```python
from build123d import *

# Parameters (mm, degrees)
SKETCH3_W          = 81.788
SKETCH3_H          = 40.894
SKETCH3_W_2        = 40.894
SKETCH3_H_2        = 15.748
CUT_EXTRUDE1_DEPTH = 4.7752


with BuildPart() as part:
    # Sketch1 → Revolve1 (revolve)
    with BuildSketch(Plane.XY):
        Polygon((0, 0), (0, 8.90905), (0.762, 9.67105), (4.0386, 9.67105), (4.8006, 8.90905), (5.5626, 8.90905), (5.5626, 10.2235), (13.4874, 10.2235), (13.4874, 0), align=None)
    revolve(axis=Axis((13.4874, 0, 0), (-1, 0, 0)))

    # Sketch2 → Cut-Revolve1 (revolve, cut)
    with BuildSketch(Plane.XY):
        Polygon((0, 0), (0, 4.3688), (-1.588923892, 4.3688), (12.852387191, 4.819651116), (13.4874, 5.454663925), (13.4874, 0), align=None)
    revolve(axis=Axis((13.4874, 0, 0), (-1, 0, 0)), mode=Mode.SUBTRACT)

    # Sketch3 → Cut-Extrude1 (cut)
    with BuildSketch(Plane(origin=(13.4874, 0, 0), x_dir=(0, 0, -1), z_dir=(1, 0, 0))):
        Rectangle(SKETCH3_W, SKETCH3_H)
        Rectangle(SKETCH3_W_2, SKETCH3_H_2, mode=Mode.SUBTRACT)
    extrude(amount=-CUT_EXTRUDE1_DEPTH, mode=Mode.SUBTRACT)

    # Sketch4 → Revolve2 (revolve)
    with BuildSketch(Plane.XY):
        with BuildLine():
            Line((4.64794893, 10.2235), (4.64794893, 10.139331804))
            Line((4.64794893, 10.139331804), (5.440112806, 9.347167928))
            ThreePointArc((5.440112806, 9.347167928), (5.477310245, 9.257365367), (5.440112806, 9.167562806))
            Line((5.440112806, 9.167562806), (5.1816, 8.90905))
            Line((5.1816, 8.90905), (4.8006, 8.90905))
            Line((4.8006, 8.90905), (4.8006, 8.65505))
            Line((4.8006, 8.65505), (5.5626, 8.65505))
            Line((5.5626, 8.65505), (5.5626, 9.51204893))
            Line((5.5626, 9.51204893), (4.85114893, 10.2235))
            Line((4.85114893, 10.2235), (4.64794893, 10.2235))
        make_face()
    revolve(axis=Axis((5.5626, 0, 0), (-1, 0, 0)))


solid = part.part
```
Work out the finished part from the listing and answer in its coordinate system (mm). A direction names the side the tool comes from. Coordinates: 2 decimals unless noted, no trailing zeros. Loops run counter-clockwise (first coordinate to the right, second up) from the corner with the lowest first, then second, coordinate; pieces in that order, holes last. Notation, with made-up numbers: (-18, 53.25) -> (6, 53.25) arc R15 ccw to (6, 81.25) -> close; hole circle Ø10 at (20, -11). An arc over 180 degrees is marked (long way). Answer as CSV lines item,"result".
Q1. A tool of negligible diameter and unlimited length cuts with its end or side. For faces 1 (the face through (8.712, 9, 0)), 2 (the face through (2.423, 9.224, -2.905)), 3 (the face through (8.712, -9, 0)), 4 (the face through (6.516, -1.002, 4.512)), from which of +Z, -Z, +X, -X, +Y, -Y can it reach the whole face along a straight path? Write none if from no direction.
Findings:
face 1,"+Z, -Z, +X, +Y"
face 2,"-X"
face 3,"+Z, -Z, +X, -Y"
face 4,"+X"
Q2. The part is cut by section C-C on x = 3. Write down the section's boundary in (y, z), and give its area (3 significant figures).
Findings:
outline,"circle Ø19.34 at (0, 0); hole circle Ø9.02 at (0, 0)"
area,"230 mm²"
Q3. The part is cut by section B-B on x = 8. Write down the section's boundary in (y, z), and give its area (3 significant figures).
Findings:
outline,"circle Ø20.45 at (0, 0); hole circle Ø9.34 at (0, 0)"
area,"260 mm²"
Q4. Each of these flat-tipped pins is pushed along its axis until it touches: pin 1 (5.5 mm diameter, centred on x = 10.5, z = -2.5, fed in from -Y); pin 2 (4 mm diameter, centred on x = 10.5, z = -1, fed in from +Y); pin 3 (1.9 mm diameter, centred on y = -9, z = -1, fed in from +X). Where does it stop, or does it pass through?
Findings:
pin 1,"stops at y = -10.22"
pin 2,"stops at y = 10.22"
pin 3,"stops at x = 8.71"
Q5. For a pull along Y with two mould halves and no side action, classify faces 5 (the face through (13.487, 5.1, -2.4)), 6 (the face through (4.994, 8.498, -2.676)), 7 (the face through (11, 7.874, 0)) as +Y half, -Y half, draft (parallel to the pull), parting line (faces both ways), or undercut.
Findings:
face 5,"draft"
face 6,"undercut"
face 7,"+Y half"
Q6. Find the intervals of material crossed by probe 1 along Z at (x, y) = (8.25, 3.5); probe 2 along Z at (x, y) = (12.25, 2.5); probe 3 along Y at (x, z) = (4.75, -6.5), in increasing order.
Findings:
probe 1,"z = -9.61 to -3.1, 3.1 to 9.61"
probe 2,"z = -9.91 to -4.1, 4.1 to 9.91"
probe 3,"y = -7.89 to -7.65, -6.17 to 6.17, 7.65 to 7.89"
